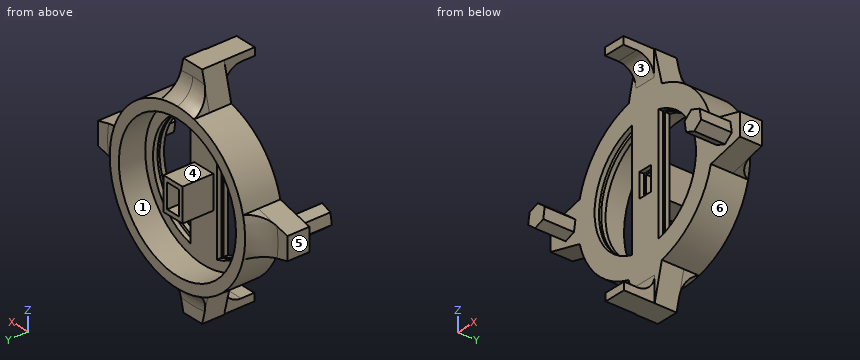
```python
from build123d import *

# Parameters (mm, degrees)
SKETCH4_R                = 17
BOSS_EXTRUDE3_DEPTH      = 6
SHELL4_T                 = 0.5
SKETCH5_W                = 3.2
SKETCH5_H                = 5.5
BOSS_EXTRUDE4_DEPTH      = 8
SHELL5_T                 = 1
BOSS_EXTRUDE6_DEPTH      = 3.5
BOSS_EXTRUDE6_DEPTH_BACK = 1.5
SKETCH7_W                = 5
SKETCH7_H                = 1.75
BOSS_EXTRUDE7_DEPTH      = 7
FILLET3_R                = 5
CUT_EXTRUDE1_DEPTH       = 5
SKETCH13_W               = 3.166032567
SKETCH13_H               = 5.463514234
CUT_EXTRUDE2_DEPTH       = 5
FILLET4_R                = 4
BOSS_EXTRUDE8_DEPTH      = 7


with BuildPart() as part:
    # Sketch4 → Boss-Extrude3 (new body)
    with BuildSketch(Plane(origin=(0, 0, 0), x_dir=(1, 0, 0), z_dir=(0, 1, 0))):
        with Locations(Location((0, -46.79046007, 0), (0, 0, 270))):
            Circle(SKETCH4_R)
    extrude(amount=BOSS_EXTRUDE3_DEPTH)

    # Shell4
    shell4_openings = [part.faces().sort_by_distance(p)[0] for p in [
        (0, 6, 46.79046007),
    ]]
    offset(amount=SHELL4_T, openings=shell4_openings, kind=Kind.INTERSECTION)

    # Sketch5 → Boss-Extrude4 (add)
    with BuildSketch(Plane(origin=(0, 0, 0), x_dir=(1, 0, 0), z_dir=(0, 1, 0))):
        with Locations((0, -46.79046007)):
            Rectangle(SKETCH5_W, SKETCH5_H)
    extrude(amount=BOSS_EXTRUDE4_DEPTH)

    # Shell5
    shell5_openings = [part.faces().sort_by_distance(p)[0] for p in [
        (0, 8, 46.79046007),
    ]]
    offset(amount=SHELL5_T, openings=shell5_openings, kind=Kind.INTERSECTION)

    # Sketch6 → Boss-Extrude6 (add, two sides: drawn at the far end of the back side and taken through both)
    with BuildSketch(Plane(origin=(0, 0, 0), x_dir=(1, 0, 0), z_dir=(0, 1, 0)).offset(-BOSS_EXTRUDE6_DEPTH_BACK)):
        with BuildLine():
            Line((-2.565219646, -72.659781842), (2.565219646, -72.659781842))
            Line((2.565219646, -72.659781842), (4.531236217, -64.726956337))
            ThreePointArc((4.531236217, -64.726956337), (0, -65.29046007), (-4.531236217, -64.726956337))
            Line((-4.531236217, -64.726956337), (-2.565219646, -72.659781842))
        make_face()
        with BuildLine():
            Line((-25.869321772, -44.225240424), (-17.936496267, -42.259223853))
            ThreePointArc((-17.936496267, -42.259223853), (-18.5, -46.79046007), (-17.936496267, -51.321696288))
            Line((-17.936496267, -51.321696288), (-25.869321772, -49.355679717))
            Line((-25.869321772, -49.355679717), (-25.869321772, -44.225240424))
        make_face()
        with BuildLine():
            Line((2.565219646, -20.921138298), (4.531236217, -28.853963803))
            ThreePointArc((4.531236217, -28.853963803), (0, -28.29046007), (-4.531236217, -28.853963803))
            Line((-4.531236217, -28.853963803), (-2.565219646, -20.921138298))
            Line((-2.565219646, -20.921138298), (2.565219646, -20.921138298))
        make_face()
        with BuildLine():
            Line((25.869321772, -49.355679717), (17.936496267, -51.321696288))
            ThreePointArc((17.936496267, -51.321696288), (18.5, -46.79046007), (17.936496267, -42.259223853))
            Line((17.936496267, -42.259223853), (25.869321772, -44.225240424))
            Line((25.869321772, -44.225240424), (25.869321772, -49.355679717))
        make_face()
    extrude(amount=BOSS_EXTRUDE6_DEPTH + BOSS_EXTRUDE6_DEPTH_BACK)

    # Sketch7 → Boss-Extrude7 (add)
    with BuildSketch(Plane(origin=(0, -1.5, 0), x_dir=(-1, 0, 0), z_dir=(0, -1, 0))):
        with Locations((0.065219646, -71.784781842)):
            Rectangle(SKETCH7_W, SKETCH7_H)
        with Locations((-0.065219646, -21.796138298)):
            Rectangle(SKETCH7_W, SKETCH7_H)
    extrude(amount=BOSS_EXTRUDE7_DEPTH)

    # Fillet3
    # the kernel refuses this fillet: 5 mm, written as the material it adds along each edge
    with BuildSketch(Plane(origin=(0, 3.5, 46.79046007), x_dir=(-0.6278344871312538, 0, -0.7783468743231616), z_dir=(0.7783468743231616, 0, -0.6278344871312538))) as fillet3_piece_1_section:
        with BuildLine():
            CenterArc((23.269696007, 5), FILLET3_R, 197.457603124, 72.542396876)
            Line((23.269696007, 0), (23.269696007, -0.1))
            Line((23.269696007, -0.1), (18.5, -0.1))
            Line((18.5, -0.1), (18.4, 0))
            ThreePointArc((18.4, 0), (18.4, 1.75), (18.40460608, 3.47))
            Line((18.40460608, 3.47), (18.5, 3.5))
        make_face()
    fillet3_piece_1 = revolve(axis=Axis((0, 3.5, 46.79046007), (0, 1, 0)), revolution_arc=102.218929963, mode=Mode.PRIVATE)
    fillet3_piece_1 = split(fillet3_piece_1, bisect_by=Plane(origin=(-20.380505818, 4.426759582, 42.864930265), z_dir=(0.24055555302697984, 0, 0.9706353722731745)), keep=Keep.TOP, mode=Mode.PRIVATE)
    fillet3_piece_1 = split(fillet3_piece_1, bisect_by=Plane(origin=(-20.380505744, 4.426759582, 50.715989893), z_dir=(0.24055555302697348, 0, -0.9706353722731761)), keep=Keep.TOP, mode=Mode.PRIVATE)
    add(fillet3_piece_1)
    with BuildSketch(Plane(origin=(0, 3.5, 46.79046007), x_dir=(0.7783347748418207, 0, 0.6278494869568123), z_dir=(0.6278494869568123, 0, -0.7783347748418207))) as fillet3_piece_2_section:
        with BuildLine():
            CenterArc((23.269696007, -5), FILLET3_R, 90, 72.542396876)
            Line((23.269696007, 0), (23.269696007, 0.1))
            Line((23.269696007, 0.1), (18.5, 0.1))
            Line((18.5, 0.1), (18.4, 0))
            ThreePointArc((18.4, 0), (18.4, -1.75), (18.40460608, -3.47))
            Line((18.40460608, -3.47), (18.5, -3.5))
        make_face()
    fillet3_piece_2 = revolve(axis=Axis((0, 3.5, 46.79046007), (0, -1, 0)), revolution_arc=51.108360804, mode=Mode.PRIVATE)
    fillet3_piece_2 = split(fillet3_piece_2, bisect_by=Plane(origin=(4.048850537, 4.426759722, 66.673369956), z_dir=(-0.970635372273176, 0, -0.24055555302697343)), keep=Keep.TOP, mode=Mode.PRIVATE)
    add(fillet3_piece_2)
    with BuildSketch(Plane(origin=(0, 3.5, 46.79046007), x_dir=(0.7783468743230912, 0, -0.6278344871313409), z_dir=(0.6278344871313409, 0, 0.7783468743230912))) as fillet3_piece_3_section:
        with BuildLine():
            CenterArc((23.269696007, 5), FILLET3_R, 197.457603124, 72.542396876)
            Line((23.269696007, 0), (23.269696007, -0.1))
            Line((23.269696007, -0.1), (18.5, -0.1))
            Line((18.5, -0.1), (18.4, 0))
            ThreePointArc((18.4, 0), (18.4, 1.75), (18.40460608, 3.47))
            Line((18.40460608, 3.47), (18.5, 3.5))
        make_face()
    fillet3_piece_3 = revolve(axis=Axis((0, 3.5, 46.79046007), (0, 1, 0)), revolution_arc=102.218929963, mode=Mode.PRIVATE)
    fillet3_piece_3 = split(fillet3_piece_3, bisect_by=Plane(origin=(3.925529805, 4.426759582, 26.409954252), z_dir=(-0.9706353722731743, 0, 0.24055555302698087)), keep=Keep.TOP, mode=Mode.PRIVATE)
    fillet3_piece_3 = split(fillet3_piece_3, bisect_by=Plane(origin=(-3.925529823, 4.426759582, 26.409954326), z_dir=(0.9706353722731764, 0, 0.2405555530269717)), keep=Keep.TOP, mode=Mode.PRIVATE)
    add(fillet3_piece_3)
    with BuildSketch(Plane(origin=(0, 3.5, 46.79046007), x_dir=(0.6278344871312218, 0, 0.7783468743231875), z_dir=(-0.7783468743231875, 0, 0.6278344871312218))) as fillet3_piece_4_section:
        with BuildLine():
            CenterArc((23.269696007, 5), FILLET3_R, 197.457603124, 72.542396876)
            Line((23.269696007, 0), (23.269696007, -0.1))
            Line((23.269696007, -0.1), (18.5, -0.1))
            Line((18.5, -0.1), (18.4, 0))
            ThreePointArc((18.4, 0), (18.4, 1.75), (18.40460608, 3.47))
            Line((18.40460608, 3.47), (18.5, 3.5))
        make_face()
    fillet3_piece_4 = revolve(axis=Axis((0, 3.5, 46.79046007), (0, 1, 0)), revolution_arc=102.218929963, mode=Mode.PRIVATE)
    fillet3_piece_4 = split(fillet3_piece_4, bisect_by=Plane(origin=(20.380505818, 4.426759582, 50.715989875), z_dir=(-0.24055555302698112, 0, -0.9706353722731741)), keep=Keep.TOP, mode=Mode.PRIVATE)
    fillet3_piece_4 = split(fillet3_piece_4, bisect_by=Plane(origin=(20.380505744, 4.426759582, 42.864930247), z_dir=(-0.24055555302697304, 0, 0.9706353722731761)), keep=Keep.TOP, mode=Mode.PRIVATE)
    add(fillet3_piece_4)
    with BuildSketch(Plane(origin=(0, 3.5, 46.79046007), x_dir=(0, 0, 1), z_dir=(1, 0, 0))) as fillet3_piece_5_section:
        with BuildLine():
            CenterArc((23.269696007, -5), FILLET3_R, 90, 72.542396876)
            Line((23.269696007, 0), (23.269696007, 0.1))
            Line((23.269696007, 0.1), (18.5, 0.1))
            Line((18.5, 0.1), (18.4, 0))
            ThreePointArc((18.4, 0), (18.4, -1.75), (18.40460608, -3.47))
            Line((18.40460608, -3.47), (18.5, -3.5))
        make_face()
    fillet3_piece_5 = revolve(axis=Axis((0, 3.5, 46.79046007), (0, -1, 0)), revolution_arc=51.108360804, mode=Mode.PRIVATE)
    fillet3_piece_5 = split(fillet3_piece_5, bisect_by=Plane(origin=(-4.04885046, 4.426759578, 66.673370268), z_dir=(0.9706353722731745, 0, -0.24055555302697917)), keep=Keep.TOP, mode=Mode.PRIVATE)
    add(fillet3_piece_5)

    # Sketch11 → Cut-Extrude1 (cut)
    with BuildSketch(Plane(origin=(0, 1, 0), x_dir=(1, 0, 0), z_dir=(0, 1, 0))):
        with BuildLine():
            Line((-3.585868376, -59.921550203), (-3.585868376, -33.501237191))
            ThreePointArc((-3.585868376, -33.501237191), (-13.861572731, -46.711393697), (-3.585868376, -59.921550203))
        make_face()
        with BuildLine():
            Line((3.585868376, -59.921550203), (3.585868376, -33.501237191))
            ThreePointArc((3.585868376, -33.501237191), (13.861572731, -46.711393697), (3.585868376, -59.921550203))
        make_face()
    extrude(amount=-CUT_EXTRUDE1_DEPTH, mode=Mode.SUBTRACT)

    # Sketch13 → Cut-Extrude2 (cut)
    with BuildSketch(Plane(origin=(0, -0.5, 0), x_dir=(1, 0, 0), z_dir=(0, 1, 0))):
        with Locations((0.016983716, -46.772217187)):
            Rectangle(SKETCH13_W, SKETCH13_H)
    extrude(amount=-CUT_EXTRUDE2_DEPTH, mode=Mode.SUBTRACT)

    # Fillet4
    fillet4_edges = [part.edges().sort_by_distance(p)[0] for p in [
        (0.065219646, -1.5, 22.671138298),
        (-0.065219646, -1.5, 70.909781842),
    ]]
    fillet(fillet4_edges, radius=FILLET4_R)

    # Sketch16 → Boss-Extrude8 (add)
    with BuildSketch(Plane(origin=(0, -1.5, 0), x_dir=(-1, 0, 0), z_dir=(0, -1, 0))):
        Polygon((19.095115037, -47.769177252), (20.96203058, -49.305079029), (23.225618307, -48.456233631), (23.622290493, -46.071486456), (21.75537495, -44.535584679), (19.491787223, -45.384430077), align=None)
        Polygon((-19.525754656, -45.384430077), (-19.12908247, -47.769177252), (-20.995998013, -49.305079029), (-23.25958574, -48.456233631), (-23.656257926, -46.071486456), (-21.789342383, -44.535584679), align=None)
    extrude(amount=BOSS_EXTRUDE8_DEPTH)


solid = part.part
```
The model under review builds one solid part; all positions refer to its coordinate system, in mm. Face numbers are marked on the shaded views. A direction names the side the tool comes from. Coordinates: 2 decimals unless noted, no trailing zeros. Order: outer loops, then holes, each group sorted by start corner. A loop starts at its lowest first (then second) coordinate and runs counter-clockwise, first axis right, second up. Notation, with made-up numbers: M 23.25,-2 L 62.25,-2 A26 cw 62.25,15 Z; hole C 76,23.5 d5. An arc over 180 degrees is marked long. One line per question, with ' | ' between items.
(1) Machinability: for the marked faces 1, 2 and 3, which of the approach directions +Z, -Z, +X, -X, +Y, -Y give a long, thin tool a straight path to every point of the face, cutting with its end or side? Answer none if there is none.
Geometry results:
face 1: +Y | face 2: +Z, -Z, +X, +Y, -Y | face 3: +X, -X, -Y
(2) Add section B-B, the plane z = 38. State how many separate pieces and enclosed holes the cut face has, then the cut area to 3 significant figures.
Geometry results:
separate pieces: 4 | enclosed holes: 0 | area: 65.7 mm²
(3) For probe 1 along Y at (x, z) = (-15, 49.5); probe 2 along X at (y, z) = (0.25, 47.5); probe 3 along Y at (x, z) = (5.5, 63.5), list the stretches that pass through material, from the lowest coordinate up. Write a range as from..to.
Geometry results:
probe 1: y = -1.5..-0.5, 0..1 | probe 2: x = -25.87..-17.49, -16.99..-13.84, -3.59..-1.6, 1.6..3.59, 13.84..16.99, 17.49..25.87 | probe 3: y = -1.5..7
(4) Add section D-D, the plane x = -8.5. Write out the cut boundary in (y, z).
Geometry results:
outline: M -1.5,30.36 L 7,30.36 L 7,33.24 L 1,33.24 L 1,35.88 L 0,35.88 L 0,32.07 L 6,32.07 L 6,31.49 L -0.5,31.49 L -0.5,35.88 L -1.5,35.88 Z; M -1.5,57.55 L -0.5,57.55 L -0.5,62.09 L 6,62.09 L 6,61.51 L 0,61.51 L 0,57.55 L 1,57.55 L 1,60.35 L 7,60.35 L 7,63.22 L -1.5,63.22 Z
(5) Add section C-C, the plane y = -2.5. Write out the cut boundary in (x, z).
Geometry results:
outline: M -23.62,46.07 L -21.76,44.54 L -19.49,45.38 L -19.1,47.77 L -20.96,49.31 L -23.23,48.46 Z; M -2.57,69.56 L 2.43,69.56 L 2.43,72.66 L -2.57,72.66 Z; M -2.43,20.92 L 2.57,20.92 L 2.57,24.03 L -2.43,24.03 Z; M 19.13,47.77 L 19.53,45.38 L 21.79,44.54 L 23.66,46.07 L 23.26,48.46 L 21,49.31 Z
(6) Add section A-A, the plane y = 2.5. Write out the cut boundary in (x, z).
Geometry results:
outline: M -25.87,44.23 L -17.94,42.26 A18.5 ccw -4.53,28.85 L -2.57,20.92 L 2.57,20.92 L 4.53,28.85 A18.5 ccw 17.94,42.26 L 25.87,44.23 L 25.87,49.36 L 17.94,51.32 A18.5 ccw 4.53,64.73 L 2.57,72.66 L -2.57,72.66 L -4.53,64.73 A18.5 ccw -17.94,51.32 L -25.87,49.36 Z; C 0,46.79 d34; M -2.6,43.04 L 2.6,43.04 L 2.6,50.54 L -2.6,50.54 Z; hole C 0,46.79 d35; hole C 0,46.79 d32; hole M -1.6,44.04 L 1.6,44.04 L 1.6,49.54 L -1.6,49.54 Z
(7) The part is to be moulded in two halves that separate along X. For the marked faces 4, 5 and 6, say which applies: +X half, -X half, draft (parallel to the pull), parting line (faces both ways), or undercut.
Geometry results:
face 4: undercut | face 5: -X half | face 6: +X half
(8) Insertion check: pin 1 (4 mm diameter, centred on y = -2, z = 56.5, fed in from -X); pin 2 (1.5 mm diameter, centred on x = -11, y = 4, fed in from -Z); pin 3 (1 mm diameter, centred on x = 0.5, y = 5, fed in from -Z). Each pin has a flat end and moves straight along its axis. Give the tip position at first contact, or say it passes through.
Geometry results:
pin 1: stops at x = -16.79 | pin 2: stops at z = 31.39 | pin 3: stops at z = 26.53
